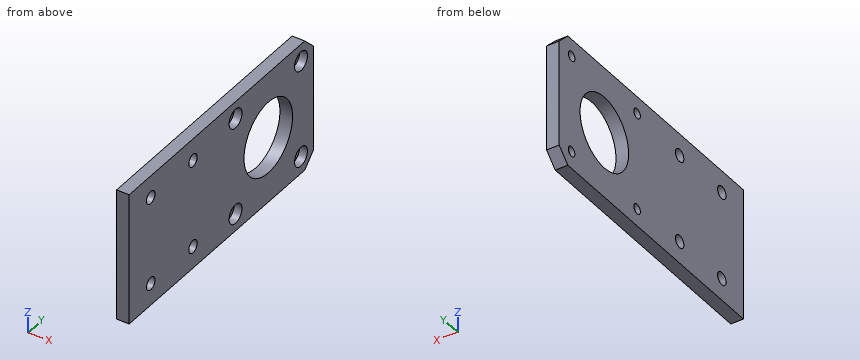
from build123d import *

# Parameters (mm, degrees)
CROQUIS1_W              = 42
CROQUIS1_H              = 87.25
SALIENTE_EXTRUIR1_DEPTH = 4
CROQUIS2_R              = 1.55
CROQUIS2_R_2            = 11.5
CORTAR_EXTRUIR1_DEPTH   = 5
CROQUIS3_R              = 2
CORTAR_EXTRUIR2_DEPTH   = 5
CHAFL_N1_SIZE           = 4.1
CROQUIS8_R              = 3.05
CORTAR_EXTRUIR3_DEPTH   = 2.5


with BuildPart() as part:
    # Croquis1 → Saliente-Extruir1 (new body)
    with BuildSketch(Plane(origin=(0, 0, 0), x_dir=(0, 0, -1), z_dir=(1, 0, 0))):
        Rectangle(CROQUIS1_W, CROQUIS1_H)
    extrude(amount=SALIENTE_EXTRUIR1_DEPTH)

    # Croquis2 → Cortar-Extruir1 (cut, through all)
    with BuildSketch(Plane(origin=(4, 0, 0), x_dir=(0, 0, -1), z_dir=(1, 0, 0))):
        with Locations((-15.5, 37.745)):
            Circle(CROQUIS2_R)
        with Locations((15.5, 37.745)):
            Circle(CROQUIS2_R)
        with Locations((15.5, 6.745)):
            Circle(CROQUIS2_R)
        with Locations((-15.5, 6.745)):
            Circle(CROQUIS2_R)
        with Locations((0, 22.245)):
            Circle(CROQUIS2_R_2)
    extrude(amount=-CORTAR_EXTRUIR1_DEPTH, mode=Mode.SUBTRACT)

    # Croquis3 → Cortar-Extruir2 (cut, through all)
    with BuildSketch(Plane(origin=(4, 0, 0), x_dir=(0, 0, -1), z_dir=(1, 0, 0))):
        with Locations((-14, -13.405)):
            Circle(CROQUIS3_R)
        with Locations((14, -13.405)):
            Circle(CROQUIS3_R)
        with Locations((-14, -33.405)):
            Circle(CROQUIS3_R)
        with Locations((14, -33.405)):
            Circle(CROQUIS3_R)
    extrude(amount=-CORTAR_EXTRUIR2_DEPTH, mode=Mode.SUBTRACT)

    # Chaflán1
    chafl_n1_edges = [part.edges().sort_by_distance(p)[0] for p in [
        (2, 43.625, 21),
        (2, 43.625, -21),
    ]]
    chamfer(chafl_n1_edges, length=CHAFL_N1_SIZE)

    # Croquis8 → Cortar-Extruir3 (cut)
    with BuildSketch(Plane(origin=(4, 0, 0), x_dir=(0, 0, -1), z_dir=(1, 0, 0))):
        with Locations((15.5, 37.745)):
            Circle(CROQUIS8_R)
        with Locations((-15.5, 37.745)):
            Circle(CROQUIS8_R)
        with Locations((-15.5, 6.745)):
            Circle(CROQUIS8_R)
        with Locations((15.5, 6.745)):
            Circle(CROQUIS8_R)
    extrude(amount=-CORTAR_EXTRUIR3_DEPTH, mode=Mode.SUBTRACT)


solid = part.part
Part model, mm, in its own coordinate system. Coordinates: 2 decimals unless noted, no trailing zeros. Order: outer loops, then holes, each group sorted by start corner. A loop starts at its lowest first (then second) coordinate and runs counter-clockwise, first axis right, second up. Notation, with made-up numbers: (82, 59.25) - (105, 59.25) arc R27 ccw to (105, 80.25) - close; hole circle Ø6 at (-24, 1). An arc over 180 degrees is marked (long way). Use CSV: the item, a comma, the result in double quotes.
Item 1: Saw through at C-C on z = -9.5. Give the cut face in (x, y) (3 decimals).
Solved:
outline,"(0, -43.625) - (4, -43.625) - (4, 15.764) - (0, 15.764) - close; (0, 28.726) - (4, 28.726) - (4, 43.625) - (0, 43.625) - close"
Item 2: Drop flat-ended pins along their axis: P1, Ø7, axis at y = 37.745, z = -15.5, coming from the +X side; P2, Ø1.8, axis at y = 37, z = 16, coming from the +X side. Give the stop position or say it passes through.
Solved:
P1,"stops at x = 4"
P2,"stops at x = 1.5"
Item 3: Probe probe 1 along Y at (x, z) = (2.8, 15.5) (3 decimals); probe 2 along Z at (x, y) = (0.5, 37); probe 3 along Y at (x, z) = (0.25, 2) (3 decimals). List the from-to ranges inside material, lowest first.
Solved:
probe 1,"y = -43.625 to -34.728, -32.082 to -14.728, -12.082 to 3.695, 9.795 to 34.695, 40.795 to 43.625"
probe 2,"z = -21 to -16.86, -14.14 to 14.14, 16.86 to 21"
probe 3,"y = -43.625 to 10.92, 33.57 to 43.625"
Item 4: Saw through at A-A on z = 0. Give the cut face in (x, y) (3 decimals).
Solved:
outline,"(0, -43.625) - (4, -43.625) - (4, 10.745) - (0, 10.745) - close; (0, 33.745) - (4, 33.745) - (4, 43.625) - (0, 43.625) - close"
Item 5: Saw through at B-B on x = 2.1. Give the number of separate pieces and of enclosed holes in the cut face, and give its area (3 significant figures).
Solved:
separate pieces,"1"
enclosed holes,"9"
area,"3,070 mm²"
